Model file for the job. Use its own axes, mm. Coordinates: 2 decimals unless noted, no trailing zeros. Order: outer loops, then holes, each group sorted by start corner. A loop starts at its lowest first (then second) coordinate and runs counter-clockwise, first axis right, second up.
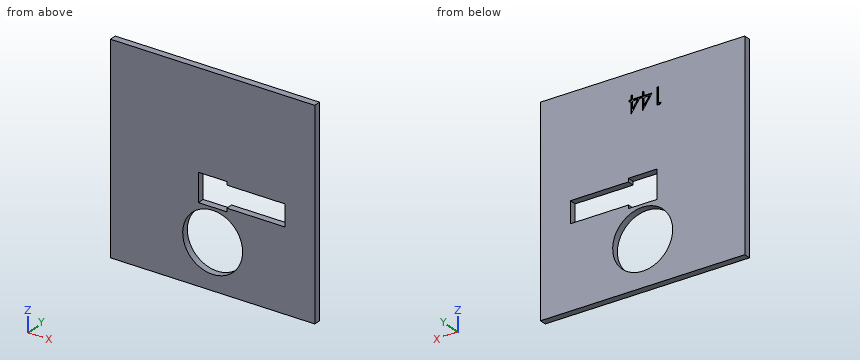
from build123d import *

# Parameters (mm, degrees)
SKETCH1_W           = 180
SKETCH1_H           = 180
SKETCH1_R           = 26.4
BOSS_EXTRUDE2_DEPTH = 6
CUT_EXTRUDE1_DEPTH  = 10
CUT_EXTRUDE2_DEPTH  = 1


with BuildPart() as part:
    # Sketch1 → Boss-Extrude2 (new body)
    with BuildSketch(Plane(origin=(0, 0, 0), x_dir=(1, 0, 0), z_dir=(0, 1, 0))):
        Rectangle(SKETCH1_W, SKETCH1_H)
        with Locations(Location((0, 50, 0), (0, 0, 270))):
            Circle(SKETCH1_R, mode=Mode.SUBTRACT)
    extrude(amount=BOSS_EXTRUDE2_DEPTH)

    # Sketch2 → Cut-Extrude1 (cut)
    with BuildSketch(Plane(origin=(0, 6, 0), x_dir=(1, 0, 0), z_dir=(0, 1, 0))):
        Polygon((-12.5, 21.1), (12.5, 21.1), (12.5, 18.1), (63.71, 18.1), (63.71, -0.9), (12.5, -0.9), (12.5, -3.9), (-12.5, -3.9), align=None)
    extrude(amount=-CUT_EXTRUDE1_DEPTH, mode=Mode.SUBTRACT)

    # Sketch3 → Cut-Extrude2 (cut)
    # profile 1 of 3: a face of its own
    with BuildSketch(Plane(origin=(0, 6, 0), x_dir=(1, 0, 0), z_dir=(0, 1, 0))):
        Polygon((-15.459341638, -56.364917997), (-12.685904138, -56.364917997), (-12.685904138, -71.364917997), (-14.032057985, -71.364917997), (-14.032057985, -57.903379535), (-16.339750292, -57.903379535), align=None)
    # profile 2 of 3: a face of its own
    with BuildSketch(Plane(origin=(0, 6, 0), x_dir=(1, 0, 0), z_dir=(0, 1, 0))):
        Polygon((-0.190110869, -55.980302612), (0.083326631, -55.980302612), (0.083326631, -66.364917997), (1.814095862, -66.364917997), (1.814095862, -67.903379535), (0.083326631, -67.903379535), (0.083326631, -71.364917997), (-1.262827215, -71.364917997), (-1.262827215, -67.903379535), (-8.378211831, -67.903379535), align=None)
        Polygon((-1.262827215, -66.364917997), (-1.262827215, -59.85049492), (-5.733981062, -66.364917997), align=None, mode=Mode.SUBTRACT)
    # profile 3 of 3: a face of its own
    with BuildSketch(Plane(origin=(0, 6, 0), x_dir=(1, 0, 0), z_dir=(0, 1, 0))):
        Polygon((10.0791199, -55.980302612), (10.3525574, -55.980302612), (10.3525574, -66.364917997), (12.083326631, -66.364917997), (12.083326631, -67.903379535), (10.3525574, -67.903379535), (10.3525574, -71.364917997), (9.006403554, -71.364917997), (9.006403554, -67.903379535), (1.891018938, -67.903379535), align=None)
        Polygon((9.006403554, -66.364917997), (9.006403554, -59.85049492), (4.535249708, -66.364917997), align=None, mode=Mode.SUBTRACT)
    extrude(amount=-CUT_EXTRUDE2_DEPTH, mode=Mode.SUBTRACT)


solid = part.part
Q1. Cut at B-B, the plane x = 29.5. List the corners of the cut face in (y, z), plus the area to 3 significant figures.
Established:
outline: (0, -90) - (6, -90) - (6, -18.1) - (0, -18.1) - close; (0, 0.9) - (6, 0.9) - (6, 90) - (0, 90) - close
area: 966 mm2
Q2. Probe line 1 (X direction, y = 2.7, z = -50); line 2 (Z direction, x = -3, y = 3.5); line 3 (X direction, y = 3.45, z = -70.5). List the from-to ranges inside material, lowest first.
Established:
line 1: x = -90 to -26.4, 26.4 to 90
line 2: z = -90 to -76.23, -23.77 to -21.1, 3.9 to 90
line 3: x = -90 to -16.63, 16.63 to 90
Q3. Cut at A-A, the plane z = -50. List the corners of the cut face in (x, y).
Established:
outline: (-90, 0) - (-26.4, 0) - (-26.4, 6) - (-90, 6) - close; (26.4, 0) - (90, 0) - (90, 6) - (26.4, 6) - close
Q4. Cut at C-C, the plane y = 1.65. List the corners of the cut face in (x, z), plus the area to 3 significant figures.
Established:
outline: (-90, -90) - (90, -90) - (90, 90) - (-90, 90) - close; hole circle Ø52.8 at (0, -50); hole (-12.5, -21.1) - (12.5, -21.1) - (12.5, -18.1) - (63.71, -18.1) - (63.71, 0.9) - (12.5, 0.9) - (12.5, 3.9) - (-12.5, 3.9) - close
area: 28,600 mm2
